```python
from build123d import *

# Parameters (mm, degrees)
F0_W     = 100
F0_H     = 33
F0_W_2   = 84.051668
F0_H_2   = 19.84357
F0_R     = 2
F1_DEPTH = 4
F2_DEPTH = 10
F3_R     = 5.08


with BuildPart() as f1:
    # F0 (on Top) → F1 (new body)
    with BuildSketch(Plane.XY):
        Rectangle(F0_W, F0_H)
        Rectangle(F0_W_2, F0_H_2, mode=Mode.SUBTRACT)
        Rectangle(F0_W_2, F0_H_2)
        with Locations((-33.341493, 0)):
            Circle(F0_R, mode=Mode.SUBTRACT)
        with Locations((32.065969, 0)):
            Circle(F0_R, mode=Mode.SUBTRACT)
    extrude(amount=F1_DEPTH)

    # F0 (on Top) → F2 (join)
    with BuildSketch(Plane.XY):
        Rectangle(F0_W, F0_H)
        Rectangle(F0_W_2, F0_H_2, mode=Mode.SUBTRACT)
    extrude(amount=F2_DEPTH)

    # F3
    f3_edges = [f1.edges().sort_by_distance(p)[0] for p in [
        (-50, 0, 10),
        (50, 0, 10),
    ]]
    fillet(f3_edges, radius=F3_R)


solid = f1.part
```
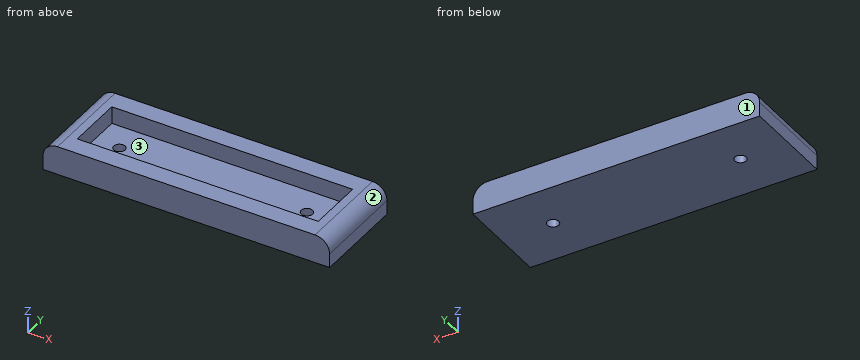
CAD build for the part. Positions are in the model's coordinates, mm. Face numbers are marked on the shaded views. Round coordinates to 2 decimals unless told otherwise and drop trailing zeros. Loops run counter-clockwise (first coordinate to the right, second up) from the corner with the lowest first, then second, coordinate; pieces in that order, holes last. Notation, with made-up numbers: (-1.75, -40) - (56.25, -40) arc R15 cw to (56.25, -26) - close; hole circle Ø3 at (17, 55.25). An arc over 180 degrees is marked (long way). Return JSON: item names as keys, results as strings. Group by question number.
Q1. Two-plate mould, pull along Y, no slides. Class the marked faces 1, 2 and 3: +Y half, -Y half, draft (parallel to the pull), parting line (faces both ways), or undercut.
Q2. Band-saw the part on C-C on x = 16. Give the cut face in (y, z).
Q3. Band-saw the part on A-A on y = 0. Give the cut face in (x, z), plus the area to 3 significant figures.
Q4. Band-saw the part on B-B on z = 6.5. Give the cut face in (x, y).
Q5. Flat gauge pins, fed straight in: pin 1 Ø3.5 at (x, y) = (-33.34, 0) entering from -Z; pin 2 Ø1.8 at (y, z) = (-3, 6) entering from +X; pin 3 Ø1 at (y, z) = (12.5, 9) entering from +X; pin 4 Ø12 at (x, y) = (11.5, -1) entering from +Z. Where does each tip first touch, or does it go through?
Q6. Drill centre lines: line 1 along Y through (x, z) = (22, 9.25); line 2 along Z through (x, y) = (-19.5, -7); line 3 along X through (y, z) = (1, 9). Where is each one in solid material? Low to high. Write a range as [from, to].
Solutions:
{
 "1": {"face 1": "+Y half", "face 2": "draft", "face 3": "undercut"},
 "2": {"outline": "(-16.5, 0) - (16.5, 0) - (16.5, 10) - (9.92, 10) - (9.92, 4) - (-9.92, 4) - (-9.92, 10) - (-16.5, 10) - close"},
 "3": {"outline": "(-50, 0) - (-35.34, 0) - (-35.34, 4) - (-42.03, 4) - (-42.03, 10) - (-44.92, 10) arc R5.08 ccw to (-50, 4.92) - close; (-31.34, 0) - (30.07, 0) - (30.07, 4) - (-31.34, 4) - close; (34.07, 0) - (50, 0) - (50, 4.92) arc R5.08 ccw to (44.92, 10) - (42.03, 10) - (42.03, 4) - (34.07, 4) - close", "area": "453 mm^2"},
 "4": {"outline": "(-49.75, -16.5) - (49.75, -16.5) - (49.75, 16.5) - (-49.75, 16.5) - close; hole (-42.03, -9.92) - (42.03, -9.92) - (42.03, 9.92) - (-42.03, 9.92) - close"},
 "5": {"pin 1": "passes through", "pin 2": "stops at x = 50", "pin 3": "stops at x = 48.52", "pin 4": "stops at z = 4"},
 "6": {"line 1": "y = [-16.5, -9.92], [9.92, 16.5]", "line 2": "z = [0, 4]", "line 3": "x = [-47.95, -42.03], [42.03, 47.95]"}
}
